from build123d import *

# Parameters (mm, degrees)
PUSHER_BASE_DEPTH   = 15
SKETCH3_R           = 1.95
SCREW_HOLE_DEPTH    = 7.5
SKETCH6_W           = 7.5
SKETCH6_H           = 30.25
PUSHER_HEAD_DEPTH   = 3.75
FILLET1_R           = 2
SKETCH9_W           = 40
SKETCH9_H           = 10
BOSS_EXTRUDE1_DEPTH = 7.5
SKETCH10_W          = 92.5
SKETCH10_H          = 4.5
BOSS_EXTRUDE2_DEPTH = 7.5
FILLET7_R           = 10
FILLET8_R           = 5
FILLET9_START       = 44.416899441
FILLET9_DEPTH       = 7.5
CUT_EXTRUDE1_DEPTH  = 10
SKETCH13_W          = 31.257668492
SKETCH13_H          = 16.460534108
CUT_EXTRUDE2_DEPTH  = 40


with BuildPart() as part:
    # Sketch1 → pusher base (new body)
    with BuildSketch(Plane.XY):
        Polygon((59.166899441, -45.877477752), (51.666899441, -45.877477752), (44.666899441, -45.877477752), (37.166899441, -45.877477752), (37.166899441, -69.377477752), (41.916899441, -69.377477752), (41.916899441, -64.127477752), (54.416899441, -64.127477752), (54.416899441, -69.377477752), (59.166899441, -69.377477752), align=None)
        with BuildLine():
            Line((48.279417247, -51.877477752), (48.054381634, -51.877477752))
            ThreePointArc((48.054381634, -51.877477752), (39.166899441, -50.877477752), (48.054381634, -49.877477752))
            Line((48.054381634, -49.877477752), (48.279417247, -49.877477752))
            ThreePointArc((48.279417247, -49.877477752), (57.166899441, -50.877477752), (48.279417247, -51.877477752))
        make_face(mode=Mode.SUBTRACT)
    extrude(amount=PUSHER_BASE_DEPTH)

    # Sketch3 → screw hole (cut)
    with BuildSketch(Plane.XZ.offset(64.127477752)):
        with Locations(Location((48.166899441, 7.5, 0), (0, 0, 270))):
            Circle(SKETCH3_R)
    extrude(amount=-SCREW_HOLE_DEPTH, mode=Mode.SUBTRACT)

    # Sketch6 → pusher head (add, symmetric)
    with BuildSketch(Plane.XY.offset(7.5)):
        with Locations((48.166899441, -30.752477752)):
            Rectangle(SKETCH6_W, SKETCH6_H)
    extrude(amount=PUSHER_HEAD_DEPTH, both=True)

    # Fillet1
    # the kernel refuses this fillet: 2 mm, written as the material it takes off along each edge
    with BuildSketch(Plane(origin=(64.166899441, -45.877477752, 0), x_dir=(0, -1, 0), z_dir=(-1, 0, 0)), Plane(origin=(32.166899441, -45.877477752, 15), x_dir=(0, -1, 0), z_dir=(1, 0, 0))) as fillet1_piece_1:
        with BuildLine():
            CenterArc((FILLET1_R, FILLET1_R), FILLET1_R, 180, 90)
            Line((0, FILLET1_R), (0, 0))
            Line((0, 0), (FILLET1_R, 0))
        make_face()
    extrude(amount=32, mode=Mode.SUBTRACT)

    # Sketch9 → Boss-Extrude1 (add)
    with BuildSketch(Plane(origin=(51.916899441, 0, 0), x_dir=(0, 0, -1), z_dir=(1, 0, 0))):
        with Locations((16.25, -20.627477752)):
            Rectangle(SKETCH9_W, SKETCH9_H)
    extrude(amount=-BOSS_EXTRUDE1_DEPTH)

    # Sketch10 → Boss-Extrude2 (add)
    with BuildSketch(Plane(origin=(0, 0, -36.25), x_dir=(-1, 0, 0), z_dir=(0, 0, -1))):
        with Locations((1.833100559, -23.377477752)):
            Rectangle(SKETCH10_W, SKETCH10_H)
    extrude(amount=-BOSS_EXTRUDE2_DEPTH)

    # Fillet7
    fillet7_edges = [part.edges().sort_by_distance(p)[0] for p in [
        (48.166899441, -15.627477752, 11.25),
    ]]
    fillet(fillet7_edges, radius=FILLET7_R)

    # Fillet8
    fillet8_edges = [part.edges().sort_by_distance(p)[0] for p in [
        (-48.083100559, -23.377477752, -36.25),
        (48.166899441, -25.627477752, 3.75),
        (51.916899441, -20.627477752, -36.25),
    ]]
    fillet(fillet8_edges, radius=FILLET8_R)

    # Fillet9: read off the stored shape, not the designer's step
    # Fillet9 outline → Fillet9 (add)
    with BuildSketch(Plane.YZ.offset(FILLET9_START)):
        with BuildLine():
            ThreePointArc((-45.877477752, 2), (-45.935475959, 1.521848316), (-46.106106786, 1.071428571))
            ThreePointArc((-46.106106786, 1.071428571), (-44.265425216, 3.02826734), (-41.677679368, 3.75))
            Line((-41.677679368, 3.75), (-45.877477752, 3.75))
            Line((-45.877477752, 3.75), (-45.877477752, 2))
        make_face()
        with BuildLine():
            Line((-45.877477752, 13), (-45.877477752, 11.25))
            Line((-45.877477752, 11.25), (-41.677679368, 11.25))
            ThreePointArc((-41.677679368, 11.25), (-44.265425216, 11.97173266), (-46.106106785, 13.928571429))
            ThreePointArc((-46.106106785, 13.928571429), (-45.935475959, 13.478151684), (-45.877477752, 13))
        make_face()
    extrude(amount=FILLET9_DEPTH)

    # Sketch12 → Cut-Extrude1 (cut)
    with BuildSketch(Plane.ZY.offset(-44.416899441)):
        with BuildLine():
            ThreePointArc((5.858454214, -30.752477752), (6.858454214, -31.752477752), (5.858454214, -32.752477752))
            Line((5.858454214, -32.752477752), (3.75, -32.752477752))
            Line((3.75, -32.752477752), (3.75, -45.877477752))
            Line((3.75, -45.877477752), (11.25, -45.877477752))
            Line((11.25, -45.877477752), (11.25, -32.752477752))
            Line((11.25, -32.752477752), (9.141545786, -32.752477752))
            ThreePointArc((9.141545786, -32.752477752), (8.141545786, -31.752477752), (9.141545786, -30.752477752))
            ThreePointArc((9.141545786, -30.752477752), (10.09823306, -29.752477752), (9.141545786, -28.752477752))
            Line((9.141545786, -28.752477752), (5.858454214, -28.752477752))
            ThreePointArc((5.858454214, -28.752477752), (4.90176694, -29.752477752), (5.858454214, -30.752477752))
        make_face()
    extrude(amount=-CUT_EXTRUDE1_DEPTH, mode=Mode.SUBTRACT)


with BuildPart() as cut_extrude1_piece_1:
    # of the separate pieces the step leaves, piece 1, a body of its own (cut_extrude1_pieces)
    add(part.part.solids().sort_by_distance((44.416899441, -30.627477752, 3.75))[0])


with BuildPart() as cut_extrude1_piece_2:
    # of the separate pieces the step leaves, piece 2, a body of its own (cut_extrude1_pieces)
    add(part.part.solids().sort_by_distance((44.416899441, -45.877477752, 11.25))[0])

    # Sketch13 → Cut-Extrude2 (cut)
    with BuildSketch(Plane.XZ.offset(32.752477752)):
        with Locations((47.849248082, 8.230267054)):
            Rectangle(SKETCH13_W, SKETCH13_H)
    extrude(amount=CUT_EXTRUDE2_DEPTH, mode=Mode.SUBTRACT)


solid = cut_extrude1_piece_1.part
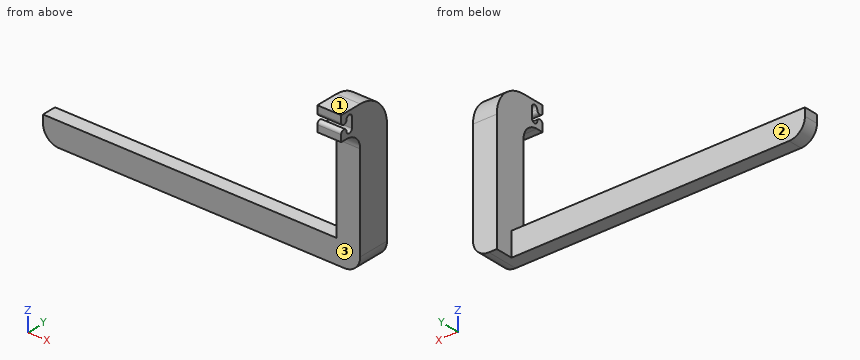
For this review, take the finished solid that the model builds, in its own axes (mm). Face numbers are marked on the shaded views. A direction names the side the tool comes from. Round coordinates to 2 decimals unless told otherwise and drop trailing zeros. Loops run counter-clockwise (first coordinate to the right, second up) from the corner with the lowest first, then second, coordinate; pieces in that order, holes last. Notation, with made-up numbers: (80.25, 37) - (98.25, 37) arc R23 ccw to (98.25, 54) - close; hole circle Ø9 at (78, 38.5). An arc over 180 degrees is marked (long way). One line per item, written item: value. Start each with the question number.
Item 1: Take a section at C-C (y = -19.5). Give the boundary of the cut face in (x, z).
Item 2: Take a section at B-B (z = -17.5). Give the boundary of the cut face in (x, y), plus the area to 3 significant figures.
Item 3: For the marked faces 1, 2 and 3, list the 3-axis set-ups (+Z, -Z, +X, -X, +Y, -Y) from which the entire face can be reached by the end or side of a thin tool; tool diameter is ignored.
Item 4: For L1, parallel to Z at x = 4, y = -25; L2, parallel to X at y = -20.75, z = -31; L3, parallel to Y at x = 46.5, z = -34, list the stretches that pass through material, from the lowest coordinate up.
Item 5: Clearance check with flat-ended pins moving along their axes: pin 1 Ø8 at (x, z) = (12, -34) entering from +Y; pin 2 Ø8 at (x, y) = (16, -27.5) entering from +Z; pin 3 Ø8.5 at (y, z) = (-23.5, -7.5) entering from -X. State where each tip first meets the part, or that it passes through.
Item 6: Take a section at A-A (x = -23.5). Give the boundary of the cut face in (y, z), plus the area to 4 significant figures.
Answer below:
1. outline: (44.42, -36.25) - (46.92, -36.25) arc R5 ccw to (51.92, -31.25) - (51.92, 9.15) - (44.42, 9.15) - close
2. outline: (44.42, -25.63) - (51.92, -25.63) - (51.92, -15.63) - (44.42, -15.63) - close
2. area: 75.0 mm2
3. face 1: +Z, +X, -X, +Y, -Y
3. face 2: +Z, -Z, -X, +Y
3. face 3: -Z, +X, -X, -Y
4. L1: z = -36.25 to -28.75
4. L2: x = 44.42 to 51.92
4. L3: y = -25.63 to -15.63
5. pin 1: stops at y = -21.13
5. pin 2: stops at z = -28.75
5. pin 3: stops at x = 44.42
6. outline: (-25.63, -36.25) - (-21.13, -36.25) - (-21.13, -28.75) - (-25.63, -28.75) - close
6. area: 33.75 mm2
